The model under review builds one solid part; all positions refer to its coordinate system, in mm. A direction names the side the tool comes from. Coordinates: 2 decimals unless noted, no trailing zeros. Write each loop counter-clockwise with the first axis right and the second up, starting at its lowest first coordinate (ties: lowest second). Pieces come first, ordered by that corner, then holes.
1) Add section B-B, the plane y = 9. State the section outline as (x, z) points.
2) Add section C-C, the plane x = 0. State the section outline as (y, z) points.
3) Add section A-A, the plane x = -31.5. State the section outline as (y, z) points.
4) For P1, Ø2, axis at x = -28.5, z = 6.5, coming from the +Y side; P2, Ø4, axis at x = 37, z = -17, coming from the -Y side; P3, Ø5, axis at y = 11, z = 2.5, coming from the +X side; P4, Ø1, axis at y = 41, z = -39, coming from the -X side, all flat-tipped, find the tip position at first contact; note any pin that passes through.
5) Add section D-D, the plane z = 0. State the section outline as (x, y) points, then the cut area to 3 significant figures.
6) Machinability: for faces 1 (the cylindrical face through (-49.997, 41.975, -0.509)), 2 (the cylindrical face through (36.175, 34.261, 36.091)), which of the approach directions +Z, -Z, +X, -X, +Y, -Y give a long, thin tool a straight path to every point of the face, cutting with its end or side? Answer none if there is none.
7) For line 1 (X direction, y = 37.5, z = 20.5); line 2 (Z direction, x = 0.5, y = 19); line 3 (Y direction, x = 8.5, z = 27), list the stretches that pass through material, from the lowest coordinate up.
8) Mouldability with a two-part tool opening along Z and no side actions: class faces 3 (the cylindrical face through (-48.794, 39.44, 25.379)), 4 (the cylindrical face through (-0.509, 41.975, 49.997)), 5 (the flat face through (1, 0, -1)) as released by +Z, released by -Z, zero draft, split by the parting line, or undercut.
from build123d import *

# Parameters (mm, degrees)
SKETCH1_R           = 55
BOSS_EXTRUDE1_DEPTH = 80
SHELL1_T            = -5
SKETCH2_R           = 4.1
CUT_EXTRUDE1_DEPTH  = 112.579568022


with BuildPart() as part:
    # Sketch1 → Boss-Extrude1 (new body)
    with BuildSketch(Plane(origin=(0, 0, 0), x_dir=(1, 0, 0), z_dir=(0, 1, 0))):
        with Locations(Location((0, 0, 0), (0, 0, 270))):
            Circle(SKETCH1_R)
    extrude(amount=BOSS_EXTRUDE1_DEPTH)

    # Shell1
    shell1_openings = [part.faces().sort_by_distance(p)[0] for p in [
        (0, 80, 0),
    ]]
    offset(amount=SHELL1_T, openings=shell1_openings, kind=Kind.INTERSECTION)

    # Sketch2 → Cut-Extrude1 (cut, through all)
    with BuildSketch(Plane(origin=(0, 80, 0), x_dir=(1, 0, 0), z_dir=(0, 1, 0))):
        with Locations(Location((-33.234018716, -33.234018716, 0), (0, 0, 270))):
            Circle(SKETCH2_R)
        with Locations(Location((-33.234018716, 33.234018716, 0), (0, 0, 270))):
            Circle(SKETCH2_R)
        with Locations(Location((33.234018716, 33.234018716, 0), (0, 0, 270))):
            Circle(SKETCH2_R)
        with Locations(Location((33.234018716, -33.234018716, 0), (0, 0, 270))):
            Circle(SKETCH2_R)
    extrude(amount=-CUT_EXTRUDE1_DEPTH, mode=Mode.SUBTRACT)


solid = part.part
Geometry results:
1. outline: circle Ø110 at (0, 0); hole (-37.33, -33.26) arc R4.1 ccw to (-33.26, -37.33) arc R50 ccw to (33.26, -37.33) arc R4.1 ccw to (37.33, -33.26) arc R50 ccw to (37.33, 33.26) arc R4.1 ccw to (33.26, 37.33) arc R50 ccw to (-33.26, 37.33) arc R4.1 ccw to (-37.33, 33.26) arc R50 ccw to start
2. outline: (0, -55) - (80, -55) - (80, -50) - (5, -50) - (5, 50) - (80, 50) - (80, 55) - (0, 55) - close
3. outline: (0, -45.09) - (80, -45.09) - (80, -38.83) - (5, -38.83) - (5, -36.95) - (0, -36.95) - close; (0, -29.52) - (5, -29.52) - (5, 29.52) - (0, 29.52) - close; (0, 36.95) - (5, 36.95) - (5, 38.83) - (80, 38.83) - (80, 45.09) - (0, 45.09) - close
4. P1: stops at y = 5
4. P2: stops at y = 0
4. P3: stops at x = 55
4. P4: stops at x = -39.28
5. outline: (-55, 0) - (55, 0) - (55, 80) - (50, 80) - (50, 5) - (-50, 5) - (-50, 80) - (-55, 80) - close
5. area: 1,300 mm2
6. face 1: +Y
6. face 2: +Y, -Y
7. line 1: x = -51.04 to -45.6, 45.6 to 51.04
7. line 2: z = -55 to -50, 50 to 55
7. line 3: y = 0 to 5
8. face 3: split by the parting line
8. face 4: undercut
8. face 5: zero draft
